Build history of the part. All positions in model axes, mm. Round coordinates to 2 decimals unless told otherwise and drop trailing zeros. Loops run counter-clockwise (first coordinate to the right, second up) from the corner with the lowest first, then second, coordinate; pieces in that order, holes last.
from build123d import *

# Parameters (mm, degrees)
EXTRUDE_1_DEPTH     = 2
SKETCH_4_R          = 1.5
CUT_EXTRUDE_3_DEPTH = 108.354552768
FILLET_4_R          = 1
CUT_EXTRUDE_5_DEPTH = 108.354552768
FILLET_7_R          = 3


with BuildPart() as part:
    # 草图1 → 凸台-拉伸1 (new body)
    with BuildSketch(Plane.XY):
        Polygon((39, 79.487179487), (33, 64.102564103), (33, -64.102564103), (39, -79.487179487), align=None)
        Polygon((33, -64.102564103), (8, 0), (0, -20.512820513), (31, -100), (39, -100), (39, -79.487179487), align=None)
        Polygon((-31, -100), (0, -20.512820513), (-8, 0), (-33, -64.102564103), (-39, -79.487179487), (-39, -100), align=None)
        Polygon((-33, -64.102564103), (-33, 64.102564103), (-39, 79.487179487), (-39, -79.487179487), align=None)
        Polygon((0, -20.512820513), (8, 0), (0, 20.512820513), (-8, 0), align=None)
        Polygon((8, 0), (33, 64.102564103), (39, 79.487179487), (39, 100), (31, 100), (0, 20.512820513), align=None)
        Polygon((-8, 0), (0, 20.512820513), (-31, 100), (-39, 100), (-39, 79.487179487), (-33, 64.102564103), align=None)
    extrude(amount=EXTRUDE_1_DEPTH)

    # 草图4 → 切除-拉伸3 (cut, through all)
    with BuildSketch(Plane.XY.offset(2)):
        with Locations((-35, 95)):
            Circle(SKETCH_4_R)
        with Locations(Location((-35, -95, 0), (0, 0, 180))):
            Circle(SKETCH_4_R)
        with Locations((35, -95)):
            Circle(SKETCH_4_R)
        with Locations(Location((35, 95, 0), (0, 0, 180))):
            Circle(SKETCH_4_R)
    extrude(amount=-CUT_EXTRUDE_3_DEPTH, mode=Mode.SUBTRACT)

    # 圆角4
    fillet_4_edges = [part.edges().sort_by_distance(p)[0] for p in [
        (39, -100, 1),
        (31, -100, 1),
        (-31, -100, 1),
        (-39, -100, 1),
        (-39, 100, 1),
        (-31, 100, 1),
        (31, 100, 1),
        (39, 100, 1),
    ]]
    fillet(fillet_4_edges, radius=FILLET_4_R)

    # 草图6 → 切除-拉伸5 (cut, through all)
    with BuildSketch(Plane.XY.offset(2)):
        Polygon((-30.751704658, -85.602329726), (-30.751704658, -99.363345276), (0, -20.512820513), (30.751704658, -99.363345276), (30.751704658, -85.602329726), (0, -6.751804962), align=None)
        Polygon((30.751704658, 85.602329726), (30.751704658, 99.363345276), (0, 20.512820513), (-30.751704658, 99.363345276), (-30.751704658, 85.602329726), (0, 6.751804962), align=None)
    extrude(amount=-CUT_EXTRUDE_5_DEPTH, mode=Mode.SUBTRACT)

    # 圆角7
    fillet_7_edges = [part.edges().sort_by_distance(p)[0] for p in [
        (30.751704658, 85.602329726, 1),
        (0, 6.751804962, 1),
        (-30.751704658, 85.602329726, 1),
        (-30.751704658, 99.363345276, 1),
        (-30.751704658, -99.363345276, 1),
        (0, -6.751804962, 1),
        (30.751704658, -85.602329726, 1),
        (30.751704658, -99.363345276, 1),
        (30.751704658, 99.363345276, 1),
        (33, 64.102564103, 1),
        (33, -64.102564103, 1),
        (8, 0, 1),
        (-8, 0, 1),
        (-33, -64.102564103, 1),
        (-33, 64.102564103, 1),
        (-30.751704658, -85.602329726, 1),
    ]]
    fillet(fillet_7_edges, radius=FILLET_7_R)


solid = part.part
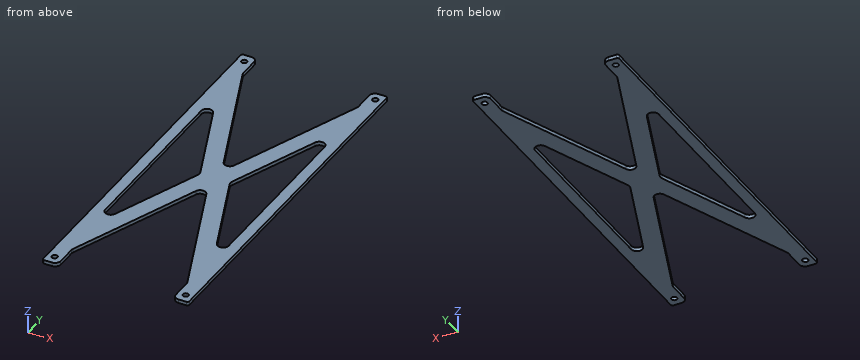
(1) Slice it at A-A on y = -61. List the corners of the cut face in (x, z), plus the area to 3 significant figures.
Responses:
outline: (-39, 0) - (-21.16, 0) - (-21.16, 2) - (-39, 2) - close; (21.16, 0) - (39, 0) - (39, 2) - (21.16, 2) - close
area: 71.4 mm2
(2) Slice it at B-B on x = -10.5. List the corners of the cut face in (y, z).
Responses:
outline: (-33.67, 0) - (-6.41, 0) - (-6.41, 2) - (-33.67, 2) - close; (6.41, 0) - (33.67, 0) - (33.67, 2) - (6.41, 2) - close
(3) Slice it at D-D on z = 1.6. Count the separate pieces of the cut face and the enclosed holes in it, plus the area to 3 significant figures.
Responses:
separate pieces: 1
enclosed holes: 6
area: 5,900 mm2
(4) Probe line 1 (Y direction, x = 35, z = 0.95); line 2 (X direction, y = -95, z = 1.6); line 3 (X direction, y = 86.5, z = 0.2). List the from-to ranges inside material, lowest first.
Responses:
line 1: y = -100 to -96.5, -93.5 to 93.5, 96.5 to 100
line 2: x = -39 to -36.5, -33.5 to -30.75, 30.75 to 33.5, 36.5 to 39
line 3: x = -39 to -30.75, 30.75 to 39
(5) Pin check, flat tip, straight feed: P1, Ø2.5, axis at x = -35, y = -95, coming from the -Z side. Stop position of the tip, or through.
Responses:
P1: passes through
(6) Slice it at C-C on y = 32.5. List the corners of the cut face in (x, z) (3 decimals).
Responses:
outline: (-39, 0) - (-33, 0) - (-33, 2) - (-39, 2) - close; (-20.675, 0) - (-10.042, 0) - (-10.042, 2) - (-20.675, 2) - close; (10.042, 0) - (20.675, 0) - (20.675, 2) - (10.042, 2) - close; (33, 0) - (39, 0) - (39, 2) - (33, 2) - close
